from build123d import *

# Parameters (mm, degrees)
SKETCH1_W           = 62
SKETCH1_H           = 50
BOSS_EXTRUDE1_DEPTH = 44
SKETCH2_R           = 10
CUT_EXTRUDE1_DEPTH  = 56
CUT_EXTRUDE2_DEPTH  = 12
CUT_EXTRUDE3_START  = -12
CUT_EXTRUDE3_DEPTH  = 12
SKETCH5_W           = 28
SKETCH5_H           = 8
CUT_EXTRUDE4_DEPTH  = 71
SKETCH6_W           = 14
SKETCH6_H           = 18
CUT_EXTRUDE5_DEPTH  = 71


with BuildPart() as part:
    # Sketch1 → Boss-Extrude1 (new body)
    with BuildSketch(Plane.XY):
        with Locations((31, 25)):
            Rectangle(SKETCH1_W, SKETCH1_H)
    extrude(amount=-BOSS_EXTRUDE1_DEPTH)

    # Sketch2 → Cut-Extrude1 (cut)
    with BuildSketch(Plane.XY):
        with Locations((31, 25)):
            Circle(SKETCH2_R)
    extrude(amount=-CUT_EXTRUDE1_DEPTH, mode=Mode.SUBTRACT)

    # Sketch3 → Cut-Extrude2 (cut)
    with BuildSketch(Plane.XY):
        with BuildLine():
            ThreePointArc((17, 25), (12.02081528, 37.02081528), (0, 42))
            Line((0, 42), (0, 8))
            ThreePointArc((0, 8), (12.02081528, 12.97918472), (17, 25))
        make_face()
        with BuildLine():
            Line((0, 8), (0, 42))
            ThreePointArc((0, 42), (-17, 25), (0, 8))
        make_face()
        with BuildLine():
            ThreePointArc((79, 25), (74.02081528, 37.02081528), (62, 42))
            Line((62, 42), (62, 8))
            ThreePointArc((62, 8), (74.02081528, 12.97918472), (79, 25))
        make_face()
        with BuildLine():
            Line((62, 8), (62, 42))
            ThreePointArc((62, 42), (45, 25), (62, 8))
        make_face()
    extrude(amount=-CUT_EXTRUDE2_DEPTH, mode=Mode.SUBTRACT)

    # Sketch4 → Cut-Extrude3 (cut)
    with BuildSketch(Plane(origin=(0, 0, -44), x_dir=(-1, 0, 0), z_dir=(0, 0, -1)).offset(CUT_EXTRUDE3_START)):
        with BuildLine():
            ThreePointArc((-62, 42), (-79, 25), (-62, 8))
            Line((-62, 8), (-62, 42))
        make_face()
        with BuildLine():
            Line((-62, 42), (-62, 8))
            ThreePointArc((-62, 8), (-49.97918472, 12.97918472), (-45, 25))
            ThreePointArc((-45, 25), (-49.97918472, 37.02081528), (-62, 42))
        make_face()
        with BuildLine():
            ThreePointArc((0, 42), (-17, 25), (0, 8))
            Line((0, 8), (0, 42))
        make_face()
        with BuildLine():
            Line((0, 42), (0, 8))
            ThreePointArc((0, 8), (12.02081528, 12.97918472), (17, 25))
            ThreePointArc((17, 25), (12.02081528, 37.02081528), (0, 42))
        make_face()
    extrude(amount=CUT_EXTRUDE3_DEPTH, mode=Mode.SUBTRACT)

    # Sketch5 → Cut-Extrude4 (cut)
    with BuildSketch(Plane.XY):
        with Locations((31, 46)):
            Rectangle(SKETCH5_W, SKETCH5_H)
    extrude(amount=-CUT_EXTRUDE4_DEPTH, mode=Mode.SUBTRACT)

    # Sketch6 → Cut-Extrude5 (cut)
    with BuildSketch(Plane.ZY):
        with Locations((-22, 25)):
            Rectangle(SKETCH6_W, SKETCH6_H)
    extrude(amount=-CUT_EXTRUDE5_DEPTH, mode=Mode.SUBTRACT)


solid = part.part
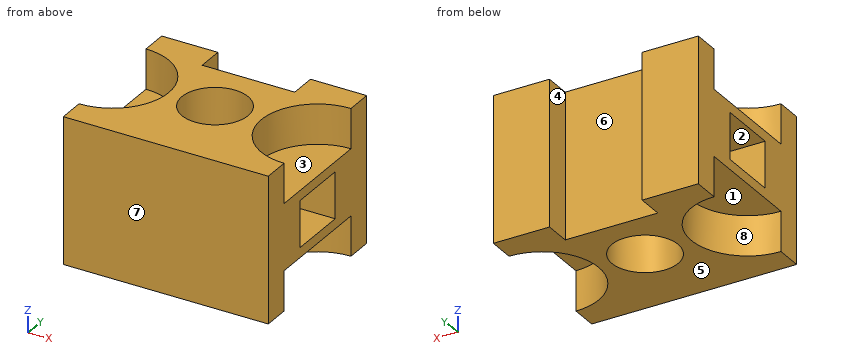
Source: CAD feature listing. Evaluate the final solid. Frame: model axes, mm. Face numbers are marked on the shaded views. A direction names the side the tool comes from. Give positions to 0.01 mm unless a question says otherwise; leave off trailing zeros. Loops run counter-clockwise (first coordinate to the right, second up) from the corner with the lowest first, then second, coordinate; pieces in that order, holes last. Notation, with made-up numbers: (64, 18.25) -> (86, 18.25) arc R14 cw to (86, 26.25) -> close; hole circle Ø4 at (82, 11). An arc over 180 degrees is marked (long way). Use a Markdown table: item, result. Add a question column.
1) Section query A-A, the plane y = 44. Return the cut outline in (x, z), then the cut area to 3 significant figures.
2) Line query: line 1 along X through (y, z) = (25, -33); line 2 along Y through (x, z) = (31, -20); line 3 along X through (y, z) = (25, -12.5). Output: solid intervals per line, ascending. Write a range as [from, to].
3) Pull-direction query (X, two-part tool) for the marked faces 6, 7 and 8; classes: +X half, -X half, draft (parallel to the pull), parting line (faces both ways), or undercut.
4) Section query B-B, the plane z = -4. Return the cut outline in (x, y).
5) Reachability of the marked faces 1, 2, 3, 4 and 5 from +Z, -Z, +X, -X, +Y, -Y: full face, straight path, thin tool, end or side. Return the list, or none.
6) Section query D-D, the plane z = -20. Return the cut outline in (x, y).
7) First-contact query: pin 1 (2 mm diameter, centred on y = 17.5, z = -7.5, fed in from -X); pin 2 (5 mm diameter, centred on x = 54, y = 24.5, fed in from +Z); pin 3 (22.5 mm diameter, centred on x = 30, z = -16, fed in from +Y). Flat tips, straight axial feed; report the tip coordinate or a pass-through.
8) Section query C-C, the plane x = 31. Return the cut outline in (y, z), then the cut area to 3 significant figures.
Numbers:
| question | item | result |
|---|---|---|
| 1 | outline | (0, -44) -> (17, -44) -> (17, 0) -> (0, 0) -> close; (45, -44) -> (62, -44) -> (62, 0) -> (45, 0) -> close |
| 1 | area | 1,500 mm2 |
| 2 | line 1 | x = [17, 21], [41, 45] |
| 2 | line 2 | y = [0, 15], [35, 42] |
| 2 | line 3 | x = [0, 21], [41, 62] |
| 3 | face 6 | undercut |
| 3 | face 7 | draft |
| 3 | face 8 | -X half |
| 4 | outline | (0, 0) -> (62, 0) -> (62, 8) arc R17 cw to (62, 42) -> (62, 50) -> (45, 50) -> (45, 42) -> (17, 42) -> (17, 50) -> (0, 50) -> (0, 42) arc R17 cw to (0, 8) -> close; hole circle Ø20 at (31, 25) |
| 5 | face 1 | -Z, -X |
| 5 | face 2 | +X, -X |
| 5 | face 3 | +Z, +X |
| 5 | face 4 | +Z, -Z, +Y |
| 5 | face 5 | -Z, +X, -X, +Y, -Y |
| 6 | outline | (0, 0) -> (62, 0) -> (62, 16) -> (35.36, 16) arc R10 cw to (26.64, 16) -> (0, 16) -> close; (0, 34) -> (26.64, 34) arc R10 cw to (35.36, 34) -> (62, 34) -> (62, 50) -> (45, 50) -> (45, 42) -> (17, 42) -> (17, 50) -> (0, 50) -> close |
| 7 | pin 1 | stops at x = 14.72 |
| 7 | pin 2 | stops at z = -12 |
| 7 | pin 3 | stops at y = 42 |
| 8 | outline | (0, -44) -> (15, -44) -> (15, 0) -> (0, 0) -> close; (35, -44) -> (42, -44) -> (42, 0) -> (35, 0) -> close |
| 8 | area | 968 mm2 |
